Read the model definition and answer for the solid it produces. Units are mm, in the model's axes. Face numbers are marked on the shaded views. Coordinates: 2 decimals unless noted, no trailing zeros. Write each loop counter-clockwise with the first axis right and the second up, starting at its lowest first coordinate (ties: lowest second). Pieces come first, ordered by that corner, then holes.
(1) Section C-C on x = 0 is taken. Write down the section's boundary in (y, z), then the cut area to 3 significant figures.
(2) The mould has two halves that part along X. Classify the marked faces 1, 2 and 3: +X half, -X half, draft (parallel to the pull), parting line (faces both ways), or undercut.
(3) Section D-D on z = -4 is taken. Write down the section's boundary in (x, y), then the cut area to 3 significant figures.
(4) Given pin 1 (1 mm diameter, centred on y = 3.5, z = 5.5, fed in from -X), flat-ended and moving along its own axis, determine where the tip first touches the part or whether it passes through.
(5) Section B-B on y = 0.85 is taken. Write down the section's boundary in (x, z).
(6) Section A-A on z = 19.5 is taken. Write down the section's boundary in (x, y).
(7) Find the intervals of material crossed by probe 1 along X at (y, z) = (1.5, 0); probe 2 along Z at (x, y) = (15.5, 1.65); probe 3 along X at (y, z) = (2.55, 19), in increasing order.
from build123d import *

# Parameters (mm, degrees)
SKETCH1_R           = 1.5
BOSS_EXTRUDE1_DEPTH = 5.08


with BuildPart() as part:
    # Sketch1 → Boss-Extrude1 (new body)
    with BuildSketch(Plane(origin=(0, 0, 0), x_dir=(1, 0, 0), z_dir=(0, 1, 0))):
        with BuildLine():
            Line((6.223, 0), (9.106543772, -18.642408089))
            ThreePointArc((9.106543772, -18.642408089), (14.180138014, -24.690685628), (21.89078133, -22.996873543))
            ThreePointArc((21.89078133, -22.996873543), (0, 31.75), (-21.89078133, -22.996873543))
            ThreePointArc((-21.89078133, -22.996873543), (-14.180138014, -24.690685628), (-9.106543772, -18.642408089))
            Line((-9.106543772, -18.642408089), (-6.223, 0))
            ThreePointArc((-6.223, 0), (0, 6.223), (6.223, 0))
        make_face()
        with Locations(Location((15.65097218, 0, 0), (0, 0, 270))):
            Circle(SKETCH1_R, mode=Mode.SUBTRACT)
        with Locations(Location((-15.65097218, 0, 0), (0, 0, 90))):
            Circle(SKETCH1_R, mode=Mode.SUBTRACT)
    extrude(amount=BOSS_EXTRUDE1_DEPTH)


solid = part.part
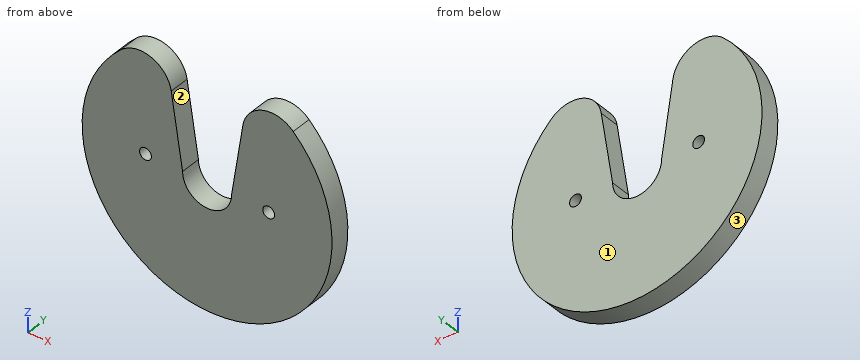
Response:
1. outline: (0, -31.75) - (5.08, -31.75) - (5.08, -6.22) - (0, -6.22) - close
1. area: 130 mm2
2. face 1: draft
2. face 2: undercut
2. face 3: parting line
3. outline: (-31.5, 0) - (-4.77, 0) - (-4.77, 5.08) - (-31.5, 5.08) - close; (4.77, 0) - (31.5, 0) - (31.5, 5.08) - (4.77, 5.08) - close
3. area: 272 mm2
4. pin 1: stops at x = -31.35
5. outline: (-21.89, 23) arc R31.75 ccw (long way) to (21.89, 23) arc R7.62 ccw to (9.11, 18.64) - (6.22, 0) arc R6.22 cw to (-6.22, 0) - (-9.11, 18.64) arc R7.62 ccw to start; hole circle Ø3 at (-15.65, 0); hole circle Ø3 at (15.65, 0)
6. outline: (-25.06, 0) - (-9.29, 0) - (-9.29, 5.08) - (-25.06, 5.08) - close; (9.29, 0) - (25.06, 0) - (25.06, 5.08) - (9.29, 5.08) - close
7. probe 1: x = -31.75 to -17.15, -14.15 to -6.22, 6.22 to 14.15, 17.15 to 31.75
7. probe 2: z = -27.71 to -1.49, 1.49 to 25.01
7. probe 3: x = -25.44 to -9.17, 9.17 to 25.44
